The model under review builds one solid part; all positions refer to its coordinate system, in mm. A direction names the side the tool comes from. Give positions to 0.01 mm unless a question says otherwise; leave off trailing zeros. Write each loop counter-clockwise with the first axis right and the second up, starting at its lowest first coordinate (ties: lowest second). Pieces come first, ordered by that corner, then holes. Notation, with made-up numbers: (85, -27.5) - (124, -27.5) arc R31 cw to (124, 11.5) - close; hole circle Ø4 at (20.25, -11.75). An arc over 180 degrees is marked (long way). Write item = value, one per line.
```python
from build123d import *

# Parameters (mm, degrees)
F1_DEPTH = 3
F0_W     = 20
F0_H     = 10
F2_DEPTH = 2
F3_W     = 45
F3_H     = 7
F3_R     = 14
F3_W_2   = 12
F3_H_2   = 9
F4_DEPTH = 15
F5_R     = 5
F6_R     = 2
F7_R     = 1


with BuildPart() as f1:
    # F0 (on Top) → F1 (new body)
    with BuildSketch(Plane.XY):
        Polygon((0, 65), (0, 0), (60, 0), (60, 10), (80, 10), (80, 0), (140, 0), (140, 65), align=None)
    extrude(amount=F1_DEPTH)

    # F1_face (on face) + F0 (on Top) → F2 (join)
    with BuildSketch(Plane(origin=(70, 33.1179775281, 3), x_dir=(1, 0, 0), z_dir=(0, 0, 1))):
        Polygon((-70, 31.8820224719), (-70, -33.1179775281), (-10, -33.1179775281), (-10, -23.1179775281), (10, -23.1179775281), (10, -33.1179775281), (70, -33.1179775281), (70, 31.8820224719), align=None)
    with BuildSketch(Plane.XY):
        with Locations((70, 5)):
            Rectangle(F0_W, F0_H)
    extrude(amount=F2_DEPTH)

    # F3 (on face) → F4 (join)
    with BuildSketch(Plane.XY):
        Polygon((61, 5), (61, 10), (60, 10), (60, 0), (80, 0), (80, 5), align=None)
        Polygon((61, 60), (135, 60), (135, 5), (80, 5), (80, 0), (140, 0), (140, 65), (0, 65), (0, 0), (60, 0), (60, 10), (61, 10), align=None)
        Polygon((10, 12), (33, 12), (33, 10), (11.25, 10), (10, 10), (10, 11.25), align=None, mode=Mode.SUBTRACT)
        with BuildLine():
            Line((43, 12.5), (50.5, 12.5))
            ThreePointArc((50.5, 12.5), (51.3838834765, 12.1338834765), (51.75, 11.25))
            ThreePointArc((51.75, 11.25), (51.3838834765, 10.3661165235), (50.5, 10))
            Line((50.5, 10), (43, 10))
            ThreePointArc((43, 10), (42.1161165235, 10.3661165235), (41.75, 11.25))
            ThreePointArc((41.75, 11.25), (42.1161165235, 12.1338834765), (43, 12.5))
        make_face(mode=Mode.SUBTRACT)
        with Locations((32.5, 23.5)):
            Rectangle(F3_W, F3_H, mode=Mode.SUBTRACT)
        with Locations((42, 46)):
            Circle(F3_R, mode=Mode.SUBTRACT)
        with Locations((16, 50.5)):
            Rectangle(F3_W_2, F3_H_2, mode=Mode.SUBTRACT)
    extrude(amount=-F4_DEPTH)

    # F5
    f5_edges = [f1.edges().sort_by_distance(p)[0] for p in [
        (98, 60, 0),
        (61, 32.5, 0),
        (98, 5, 0),
        (135, 32.5, 0),
    ]]
    fillet(f5_edges, radius=F5_R)

    # F6
    f6_edges = [f1.edges().sort_by_distance(p)[0] for p in [
        (98, 60, -15),
        (135, 32.5, -15),
        (98, 5, -15),
        (61, 32.5, -15),
        (28, 46, -15),
        (16, 55, -15),
        (10, 50.5, -15),
        (16, 46, -15),
        (22, 50.5, -15),
        (32.5, 27, -15),
        (10, 23.5, -15),
        (32.5, 20, -15),
        (55, 23.5, -15),
        (46.75, 12.5, -15),
        (21.5, 10, -15),
        (33, 11, -15),
        (21.5, 12, -15),
        (10, 11, -15),
    ]]
    fillet(f6_edges, radius=F6_R)

    # F7
    f7_edges = [f1.edges().sort_by_distance(p)[0] for p in [
        (140, 32.5, -15),
        (70, 65, -15),
        (0, 32.5, -15),
        (70, 0, -15),
        (0, 0, -5),
        (140, 0, -5),
        (140, 65, -5),
        (0, 65, -5),
    ]]
    fillet(f7_edges, radius=F7_R)


solid = f1.part
```
1. Take a section at B-B on x = 81.5. Give the boundary of the cut face in (y, z).
Findings below:
outline = (0, -14) arc R1 ccw to (1, -15) - (3, -15) arc R2 ccw to (5, -13) - (5, -5) arc R5 cw to (10, 0) - (55, 0) arc R5 cw to (60, -5) - (60, -13) arc R2 ccw to (62, -15) - (64, -15) arc R1 ccw to (65, -14) - (65, 5) - (0, 5) - close
2. Take a section at C-C on z = -8. Count the separate pieces of the cut face and the enclosed holes in it, and give its area (3 significant figures).
Findings below:
separate_pieces = 1
enclosed_holes = 6
area = 3,920 mm²
3. Take a section at A-A on z = 3.75. Give the boundary of the cut face in (x, y), and give its area (3 significant figures).
Findings below:
outline = (0, 1) arc R1 ccw to (1, 0) - (60, 0) - (60, 10) - (80, 10) - (80, 0) - (139, 0) arc R1 ccw to (140, 1) - (140, 64) arc R1 ccw to (139, 65) - (1, 65) arc R1 ccw to (0, 64) - close
area = 8,900 mm²
4. For line 1 (Y direction, x = 12, z = -8.25); line 2 (X direction, y = 23.5, z = -8.5); line 3 (Y direction, x = 26.5, z = -11.5), list the stretches that pass through material, from the lowest coordinate up. Write a range as from..to.
Findings below:
line_1 = 0..10, 12..20, 27..46, 55..65
line_2 = 0..10, 55..61, 135..140
line_3 = 0..10, 12..20, 27..65
5. Insertion check: P1, Ø4.5, axis at x = 16.5, y = 49.5, coming from the -Z side; P2, Ø7.5, axis at x = 26, y = 24, coming from the -Z side; P3, Ø1.5, axis at x = 60.5, y = 48, coming from the -Z side. Each pin has a flat end and moves straight along its axis. Give the tip position at first contact, or say it passes through.
Findings below:
P1 = 0
P2 = -14.56
P3 = -14.85
6. Draft analysis for pull direction X (two halves, no side actions). For faces 4 (the flat face through (69, 33, 5)), 5 (the flat face through (97, 60, -9)), 6 (the flat face through (140, 32, -4)), state which applies: +X half, -X half, draft (parallel to the pull), parting line (faces both ways), or undercut.
Findings below:
face_4 = draft
face_5 = undercut
face_6 = +X half
7. Machinability: for faces 1 (the flat face through (71, 65, -4)), 2 (the flat face through (70, 5, 2)), 3 (the cylindrical face through (63, 33, -1)), which of the approach directions +Z, -Z, +X, -X, +Y, -Y give a long, thin tool a straight path to every point of the face, cutting with its end or side? Answer none if there is none.
Findings below:
face_1 = +Z, -Z, +X, -X, +Y
face_2 = +Z, -Y
face_3 = -Z
